For this review, take the finished solid that the model builds, in its own axes (mm). A direction names the side the tool comes from. Give positions to 0.01 mm unless a question says otherwise; leave off trailing zeros. Loops run counter-clockwise (first coordinate to the right, second up) from the corner with the lowest first, then second, coordinate; pieces in that order, holes last. Notation, with made-up numbers: (-31.75, 52) -> (-27.75, 52) arc R27 cw to (-27.75, 75) -> close; hole circle Ø11 at (77, 71.25). An arc over 180 degrees is marked (long way). Write each question's results on one line, items separated by ' | '. Start each with the question number.
```python
from build123d import *

# Parameters (mm, degrees)
PAD018_DEPTH    = 3
PAD018_TAPER    = 14
SKETCH032_R     = 10
HOLE009_DEPTH   = 25
SKETCH034_R     = 2
PAD022_DEPTH    = 4
POCKET002_DEPTH = 4.6
POCKET002_TAPER = 15


with BuildPart() as part:
    # Sketch031 → Pad018 (new body)
    with BuildSketch(Plane.XY.offset(-4)):
        with BuildLine():
            ThreePointArc((-17.734351, 11.23491), (-16.243686, 13.811706), (-14.965, 16.5))
            Line((-14.965, 16.5), (14.965, 16.5))
            ThreePointArc((14.965, 16.5), (16.243686, 13.811706), (17.734351, 11.23491))
            ThreePointArc((12.98, -16.5), (20.691765, -3.547007), (17.734351, 11.23491))
            Line((-12.98, -16.5), (12.98, -16.5))
            ThreePointArc((-17.734351, 11.23491), (-20.691765, -3.547007), (-12.98, -16.5))
        make_face()
    extrude(amount=-PAD018_DEPTH, taper=PAD018_TAPER)

    # Sketch032 → Hole009 (cut)
    with BuildSketch(Plane.XY.offset(-4)):
        Circle(SKETCH032_R)
    extrude(amount=-HOLE009_DEPTH, mode=Mode.SUBTRACT)

    # Sketch034 → Pad022 (join)
    with BuildSketch(Plane.XY):
        with BuildLine():
            ThreePointArc((13.586881, 20.251823), (0, 30.3), (-13.586881, 20.251823))
            ThreePointArc((-17.728491, 11.256137), (-15.355357, 15.614788), (-13.586881, 20.251823))
            ThreePointArc((-17.728491, 11.256137), (-20.699674, -3.538854), (-12.982142, -16.506483))
            ThreePointArc((-6.502297, -26.893782), (-8.833051, -21.132971), (-12.982142, -16.506483))
            ThreePointArc((-6.502297, -26.893782), (0, -32.15), (6.502297, -26.893782))
            ThreePointArc((12.982142, -16.506483), (8.833051, -21.132971), (6.502297, -26.893782))
            ThreePointArc((12.982142, -16.506483), (20.699674, -3.538854), (17.728491, 11.256137))
            ThreePointArc((13.586881, 20.251823), (15.355357, 15.614788), (17.728491, 11.256137))
        make_face()
        with Locations((0, -25.5)):
            Circle(SKETCH034_R, mode=Mode.SUBTRACT)
        with Locations((-8, 21.5)):
            Circle(SKETCH034_R, mode=Mode.SUBTRACT)
        with Locations((8, 21.5)):
            Circle(SKETCH034_R, mode=Mode.SUBTRACT)
    extrude(amount=-PAD022_DEPTH)

    # Sketch035 → Pocket002 (cut)
    with BuildSketch(Plane.XY):
        with BuildLine():
            Line((-14.85, 11.05), (-14.85, -10.95))
            ThreePointArc((-14.85, -10.95), (-13.649138, -13.849138), (-10.75, -15.05))
            Line((-10.75, -15.05), (10.85, -15.05))
            ThreePointArc((10.85, -15.05), (13.678427, -13.878427), (14.85, -11.05))
            Line((14.85, -11.05), (14.85, 11.05))
            ThreePointArc((14.85, 11.05), (13.678427, 13.878427), (10.85, 15.05))
            Line((10.85, 15.05), (-10.85, 15.05))
            ThreePointArc((-10.85, 15.05), (-13.678427, 13.878427), (-14.85, 11.05))
        make_face()
    extrude(amount=-POCKET002_DEPTH, taper=POCKET002_TAPER, mode=Mode.SUBTRACT)


with BuildPart() as part_1:
    # Body010 placement: moved
    add(part.part.moved(Location((0, 0, -4))))


solid = part_1.part
```
1. Wall thickness on L1, parallel to Y at x = 8, z = -5.75; L2, parallel to Y at x = 7.5, z = -5.5; L3, parallel to Z at x = 1, y = 28.5: over which ranges is each line inside the solid? List them lowest first.
2. We need section A-A (y = 21.5). Write out the cut boundary in (x, z).
3. Draft analysis for pull direction X (two halves, no side actions). For faces 1 (the cylindrical face through (20.662, -3.752, -5.972)), 2 (the flat face through (6.1, 15.4, -4)), 3 (the cylindrical face through (6.002, 21.588, -5.972)), 4 (the cylindrical face through (-0.13, -32.15, -5.97)), state which applies: released by +X, released by -X, zero draft, split by the parting line, or undercut.
4. For pin 1 Ø13.5 at (x, y) = (4, 4.5) entering from +Z; pin 2 Ø1.5 at (y, z) = (8.5, -7.5) entering from -X; pin 3 Ø3 at (y, z) = (-21.5, -8.5) entering from +X, all flat-tipped, find the tip position at first contact; note any pin that passes through.
5. Machinability: for faces 5 (the flat face through (9, 6, -8.6)), 6 (the flat face through (0, 22, -8)), 7 (the cylindrical face through (-20.735, -3.326, -5.972)), which of the approach directions +Z, -Z, +X, -X, +Y, -Y give a long, thin tool a straight path to every point of the face, cutting with its end or side? Answer none if there is none.
6. We need section B-B (x = 0). Count the separate pieces of the cut face and the enclosed holes in it, plus the area to 3 significant figures.
Response:
1) L1: y = -22.62 to -14.58, 14.58 to 19.5, 23.5 to 27.83 | L2: y = -23.71 to -14.65, 14.65 to 19.56, 23.44 to 28.16 | L3: z = -8 to -4
2) outline: (-13.14, -8) -> (-10, -8) -> (-10, -4) -> (-13.14, -4) -> close; (-6, -8) -> (6, -8) -> (6, -4) -> (-6, -4) -> close; (10, -8) -> (13.14, -8) -> (13.14, -4) -> (10, -4) -> close
3) face 1: released by +X | face 2: zero draft | face 3: undercut | face 4: split by the parting line
4) pin 1: stops at z = -8.6 | pin 2: stops at x = -19.52 | pin 3: stops at x = 9.54
5) face 5: +Z | face 6: -Z, +X, -X, +Y | face 7: +Z, -Z, -X
6) separate pieces: 3 | enclosed holes: 0 | area: 150 mm2
